Geometry: final body of the model. Coordinates: model frame, mm. Face numbers are marked on the shaded views. A direction names the side the tool comes from. Give positions to 0.01 mm unless a question says otherwise; leave off trailing zeros. Order: outer loops, then holes, each group sorted by start corner. A loop starts at its lowest first (then second) coordinate and runs counter-clockwise, first axis right, second up. Notation, with made-up numbers: M 57.25,28 L 112.25,28 A11 ccw 112.25,36 Z; hole C 6,-18.75 d3. An arc over 180 degrees is marked long. Use CSV: the item, a comma, the result in double quotes.
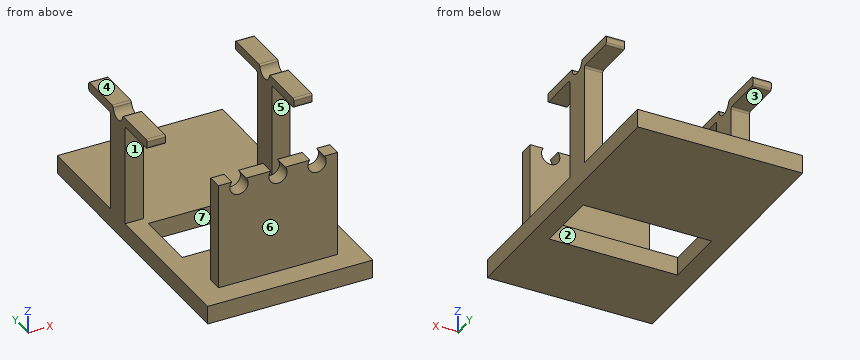
```python
from build123d import *

# Parameters (mm, degrees)
SKETCH1_W               = 125
SKETCH1_H               = 90
BOSS_EXTRUDE1_DEPTH     = 10
BOSS_EXTRUDE2_DEPTH     = 35
BOSS_EXTRUDE3_DEPTH     = 45
SKETCH11_W              = 90
SKETCH11_H              = 30
BOSS_EXTRUDE5_DEPTH     = 10
CUT_EXTRUDE2_DEPTH      = 126
CUT_EXTRUDE2_DEPTH_BACK = 126
SKETCH7_W               = 35
SKETCH7_H               = 43
SKETCH7_H_2             = 6
SKETCH7_H_3             = 1
SKETCH17_W              = 60.575148418
SKETCH17_H              = 1.596164387
SKETCH17_W_2            = 94.424851582
BOSS_EXTRUDE7_DEPTH     = 90
SKETCH18_W              = 155
SKETCH18_H              = 8.403835613
BOSS_EXTRUDE8_DEPTH     = 90
CUT_EXTRUDE3_DEPTH      = 143.324453275
CUT_EXTRUDE3_DEPTH_BACK = 143.324453275
CUT_EXTRUDE4_DEPTH      = 126
CUT_EXTRUDE4_DEPTH_BACK = 126
SKETCH21_W              = 70
SKETCH21_H              = 10
CUT_EXTRUDE5_DEPTH      = 120.085053638
CUT_EXTRUDE5_DEPTH_BACK = 120.085053638
SKETCH22_W              = 70
SKETCH22_H              = 35
SKETCH23_W              = 65
SKETCH23_H              = 8
BOSS_EXTRUDE9_DEPTH     = 58
SKETCH24_R              = 5
CUT_EXTRUDE6_DEPTH      = 29


with BuildPart() as part:
    # Sketch1 → Boss-Extrude1 (new body)
    with BuildSketch(Plane(origin=(0, 0, 0), x_dir=(0, 1, 0), z_dir=(0, 0, 1))):
        Rectangle(SKETCH1_W, SKETCH1_H)
    extrude(amount=BOSS_EXTRUDE1_DEPTH)

    # Sketch3 → Boss-Extrude2 (add, symmetric)
    with BuildSketch(Plane.YZ):
        with BuildLine():
            Line((5.916079783, 60), (7.5, 60))
            Line((7.5, 60), (29.144025452, 60))
            ThreePointArc((29.144025452, 60), (29.851132233, 59.707106781), (30.144025452, 59))
            Line((30.144025452, 59), (30.144025452, 56))
            ThreePointArc((30.144025452, 56), (29.851132233, 55.292893219), (29.144025452, 55))
            Line((29.144025452, 55), (8.5, 55))
            ThreePointArc((8.5, 55), (7.792893219, 54.707106781), (7.5, 54))
            Line((7.5, 54), (7.5, 0))
            Line((7.5, 0), (-7.5, 0))
            Line((-7.5, 0), (-7.5, 54))
            ThreePointArc((-7.5, 54), (-7.792893219, 54.707106781), (-8.5, 55))
            Line((-8.5, 55), (-29.144025452, 55))
            ThreePointArc((-29.144025452, 55), (-29.851132233, 55.292893219), (-30.144025452, 56))
            Line((-30.144025452, 56), (-30.144025452, 59))
            ThreePointArc((-30.144025452, 59), (-29.851132233, 59.707106781), (-29.144025452, 60))
            Line((-29.144025452, 60), (-7.5, 60))
            Line((-7.5, 60), (-5.916079783, 60))
            ThreePointArc((-5.916079783, 60), (-5.270582559, 59.763762616), (-4.930066486, 59.166666667))
            ThreePointArc((-4.930066486, 59.166666667), (0, 55), (4.930066486, 59.166666667))
            ThreePointArc((4.930066486, 59.166666667), (5.270582559, 59.763762616), (5.916079783, 60))
        make_face()
    extrude(amount=BOSS_EXTRUDE2_DEPTH, both=True)

    # Sketch5 → Boss-Extrude3 (add, symmetric)
    with BuildSketch(Plane.YZ):
        with BuildLine():
            ThreePointArc((-7.5, 54), (-7.792893219, 54.707106781), (-8.5, 55))
            Line((-8.5, 55), (-29.144025452, 55))
            ThreePointArc((-29.144025452, 55), (-29.851132233, 55.292893219), (-30.144025452, 56))
            Line((-30.144025452, 56), (-30.144025452, 59))
            ThreePointArc((-30.144025452, 59), (-29.851132233, 59.707106781), (-29.144025452, 60))
            Line((-29.144025452, 60), (-5.916079783, 60))
            ThreePointArc((-5.916079783, 60), (-5.270582559, 59.763762616), (-4.930066486, 59.166666667))
            ThreePointArc((-4.930066486, 59.166666667), (0, 55), (4.930066486, 59.166666667))
            ThreePointArc((4.930066486, 59.166666667), (5.270582559, 59.763762616), (5.916079783, 60))
            Line((5.916079783, 60), (29.144025452, 60))
            ThreePointArc((29.144025452, 60), (29.851132233, 59.707106781), (30.144025452, 59))
            Line((30.144025452, 59), (30.144025452, 56))
            ThreePointArc((30.144025452, 56), (29.851132233, 55.292893219), (29.144025452, 55))
            Line((29.144025452, 55), (8.5, 55))
            ThreePointArc((8.5, 55), (7.792893219, 54.707106781), (7.5, 54))
            Line((7.5, 54), (7.5, 11))
            ThreePointArc((7.5, 11), (7.792893219, 10.292893219), (8.5, 10))
            Line((8.5, 10), (-8.5, 10))
            ThreePointArc((-8.5, 10), (-7.792893219, 10.292893219), (-7.5, 11))
            Line((-7.5, 11), (-7.5, 54))
        make_face()
    extrude(amount=BOSS_EXTRUDE3_DEPTH, both=True)

    # Sketch11 → Boss-Extrude5 (add)
    with BuildSketch(Plane.XY.offset(10)):
        with Locations((0, -77.5)):
            Rectangle(SKETCH11_W, SKETCH11_H)
    extrude(amount=-BOSS_EXTRUDE5_DEPTH)

    # Sketch7 → Cut-Extrude2 (cut, two sides: drawn at the far end of the back side and taken through both)
    with BuildSketch(Plane(origin=(0, 7.5, 0), x_dir=(-1, 0, 0), z_dir=(0, 1, 0)).offset(-CUT_EXTRUDE2_DEPTH_BACK)):
        with Locations((-17.5, 32.5)):
            Rectangle(SKETCH7_W, SKETCH7_H)
        Polygon((0, 54), (0, 11), (35, 11), (35, 35), (35, 54), align=None)
        with Locations((17.5, 57)):
            Rectangle(SKETCH7_W, SKETCH7_H_2)
        with Locations((-17.5, 57)):
            Rectangle(SKETCH7_W, SKETCH7_H_2)
        with Locations((-17.5, 10.5)):
            Rectangle(SKETCH7_W, SKETCH7_H_3)
        with Locations((17.5, 10.5)):
            Rectangle(SKETCH7_W, SKETCH7_H_3)
    extrude(amount=CUT_EXTRUDE2_DEPTH + CUT_EXTRUDE2_DEPTH_BACK, mode=Mode.SUBTRACT)

    # Sketch17 → Boss-Extrude7 (add)
    with BuildSketch(Plane.YZ.offset(45)):
        with Locations((-62.212425791, -0.798082194)):
            Rectangle(SKETCH17_W, SKETCH17_H)
        with Locations((15.287574209, -0.798082194)):
            Rectangle(SKETCH17_W_2, SKETCH17_H)
    extrude(amount=-BOSS_EXTRUDE7_DEPTH)

    # Sketch18 → Boss-Extrude8 (add)
    with BuildSketch(Plane.YZ.offset(45)):
        with Locations((-15, -5.798082193)):
            Rectangle(SKETCH18_W, SKETCH18_H)
    extrude(amount=-BOSS_EXTRUDE8_DEPTH)

    # Sketch19 → Cut-Extrude3 (cut, two sides: drawn at the far end of the back side and taken through both)
    with BuildSketch(Plane.YZ.offset(45).offset(-CUT_EXTRUDE3_DEPTH_BACK)):
        with BuildLine():
            Line((-92.5, 10), (-8.5, 10))
            ThreePointArc((-8.5, 10), (-7.792893219, 10.292893219), (-7.5, 11))
            Line((-7.5, 11), (-7.5, 0))
            Line((-7.5, 0), (-92.5, 0))
            Line((-92.5, 0), (-92.5, 10))
        make_face()
        with BuildLine():
            Line((62.5, 10), (62.5, 0))
            Line((62.5, 0), (7.5, 0))
            Line((7.5, 0), (7.5, 11))
            ThreePointArc((7.5, 11), (7.792893219, 10.292893219), (8.5, 10))
            Line((8.5, 10), (62.5, 10))
        make_face()
    extrude(amount=CUT_EXTRUDE3_DEPTH + CUT_EXTRUDE3_DEPTH_BACK, mode=Mode.SUBTRACT)

    # Sketch21 → Cut-Extrude4 (cut, two sides: drawn at the far end of the back side and taken through both)
    with BuildSketch(Plane(origin=(0, 7.5, 0), x_dir=(-1, 0, 0), z_dir=(0, 1, 0)).offset(-CUT_EXTRUDE4_DEPTH_BACK)):
        with Locations((0, 5)):
            Rectangle(SKETCH21_W, SKETCH21_H)
    extrude(amount=CUT_EXTRUDE4_DEPTH + CUT_EXTRUDE4_DEPTH_BACK, mode=Mode.SUBTRACT)

    # Sketch22 → Cut-Extrude5 (cut, two sides: drawn at the far end of the back side and taken through both)
    with BuildSketch(Plane.XY.offset(-CUT_EXTRUDE5_DEPTH_BACK)):
        with Locations((0, -30)):
            Rectangle(SKETCH22_W, SKETCH22_H)
    extrude(amount=CUT_EXTRUDE5_DEPTH + CUT_EXTRUDE5_DEPTH_BACK, mode=Mode.SUBTRACT)

    # Sketch23 → Boss-Extrude9 (add)
    with BuildSketch(Plane.XY):
        with Locations((0, -76)):
            Rectangle(SKETCH23_W, SKETCH23_H)
    extrude(amount=BOSS_EXTRUDE9_DEPTH)

    # Sketch24 → Cut-Extrude6 (cut, symmetric)
    with BuildSketch(Plane.XZ.offset(80)):
        with Locations((0, 55)):
            Circle(SKETCH24_R)
        with Locations((-21.3, 55)):
            Circle(SKETCH24_R)
        with Locations((21.3, 55)):
            Circle(SKETCH24_R)
    extrude(amount=CUT_EXTRUDE6_DEPTH, both=True, mode=Mode.SUBTRACT)


solid = part.part
```
1. Section C-C, the plane y = -3. Return the cut outline in (x, z), plus the area to 3 significant figures.
Answer:
outline,"M -45,-10 L 45,-10 L 45,56 L 35,56 L 35,0 L -35,0 L -35,56 L -45,56 Z"
area,"2,020 mm2"
2. Section A-A, the plane x = 29. Return the cut outline in (y, z), plus the area to 3 significant figures.
Answer:
outline,"M -92.5,-10 L -47.5,-10 L -47.5,0 L -72,0 L -72,58 L -80,58 L -80,0 L -92.5,0 Z; M -12.5,-10 L 62.5,-10 L 62.5,0 L -12.5,0 Z"
area,"1,660 mm2"
3. Pull-direction query (Z, two-part tool) for the marked faces 1, 2, 3 and 4; classes: +Z half, -Z half, draft (parallel to the pull), parting line (faces both ways), or undercut.
Answer:
face 1,"undercut"
face 2,"draft"
face 3,"undercut"
face 4,"+Z half"
4. Section B-B, the plane z = 17. Return the cut outline in (x, y), plus the area to 3 significant figures.
Answer:
outline,"M -45,-7.5 L -35,-7.5 L -35,7.5 L -45,7.5 Z; M -32.5,-80 L 32.5,-80 L 32.5,-72 L -32.5,-72 Z; M 35,-7.5 L 45,-7.5 L 45,7.5 L 35,7.5 Z"
area,"820 mm2"
5. Reachability of the marked faces 5, 6 and 7 from +Z, -Z, +X, -X, +Y, -Y: full face, straight path, thin tool, end or side. Return the list, or none.
Answer:
face 5,"+X, -X, -Y"
face 6,"+Z, +X, -X, -Y"
face 7,"+Z, -Z"
6. Section D-D, the plane x = -21.3. Return the cut outline in (y, z), plus the area to 3 significant figures.
Answer:
outline,"M -92.5,-10 L -47.5,-10 L -47.5,0 L -72,0 L -72,50 L -80,50 L -80,0 L -92.5,0 Z; M -12.5,-10 L 62.5,-10 L 62.5,0 L -12.5,0 Z"
area,"1,600 mm2"
7. Line query: line 1 (X direction, y = -74, z = 55); line 2 (Y direction, x = -14.5, z = -6); line 3 (Z direction, x = 40, y = -15). Output: solid intervals per line, ascending.
Answer:
line 1,"-32.5 to -26.3, -16.3 to -5, 5 to 16.3, 26.3 to 32.5"
line 2,"-92.5 to -47.5, -12.5 to 62.5"
line 3,"-10 to 0, 55 to 60"
8. Pin query (flat end, axial travel): pin 1 Ø8 at (x, z) = (-41, 29) entering from +Y; pin 2 Ø13 at (x, z) = (0, 55) entering from +Y; pin 3 Ø0.9 at (x, z) = (-37.5, 57.5) entering from -Y. Return the tip coordinate at first contact, or that it passes through.
Answer:
pin 1,"y = 7.5"
pin 2,"y = -72"
pin 3,"y = -30.14"
